from build123d import *

# Parameters (mm, degrees)
SKETCH1_R           = 6.35
BOSS_EXTRUDE1_DEPTH = 17.5
CUT_EXTRUDE1_DEPTH  = 12.9
CHAMFER1_SIZE       = 2
SKETCH4_R           = 3.5
BOSS_EXTRUDE2_DEPTH = 25
SKETCH8_R           = 1.625
CUT_EXTRUDE4_DEPTH  = 30
SKETCH7_R           = 2.2
CUT_EXTRUDE3_DEPTH  = 4.5
SKETCH9_R           = 4
SKETCH9_R_2         = 1.625
BOSS_EXTRUDE3_DEPTH = 5
SKETCH11_R          = 2.75
CUT_EXTRUDE5_DEPTH  = 3
SKETCH12_R          = 1.625
CUT_EXTRUDE6_DEPTH  = 101.436547133
CUT_EXTRUDE8_REACH  = 100.805
SKETCH15_W          = 2
SKETCH15_H          = 32.561115391
SKETCH15_H_2        = 13.634806385
SKETCH16_W          = 2
SKETCH16_H          = 5.291502622
CUT_EXTRUDE9_DEPTH  = 20
CUT_EXTRUDE10_REACH = 102.437
SKETCH17_R          = 1.5
CUT_EXTRUDE11_REACH = 102.437
SKETCH18_W          = 1.2
SKETCH18_H          = 8
SKETCH19_W          = 20
SKETCH19_H          = 25
BOSS_EXTRUDE4_DEPTH = 7
CUT_EXTRUDE12_DEPTH = 35


with BuildPart() as part:
    # Sketch1 → Boss-Extrude1 (new, symmetric)
    with BuildSketch(Plane(origin=(0, 0, 0), x_dir=(0, 0, -1), z_dir=(1, 0, 0))):
        with BuildLine():
            Line((-75, -17.5), (75, -17.5))
            ThreePointArc((75, -17.5), (91.201851746, -6.614378278), (87.247448714, 12.5))
            Line((87.247448714, 12.5), (-69.247448714, 12.5))
            Line((-69.247448714, 12.5), (-69.247448714, 17.5))
            Line((-69.247448714, 17.5), (-75, 17.5))
            ThreePointArc((-75, 17.5), (-92.5, 0), (-75, -17.5))
        make_face()
        with Locations((-75, 0)):
            Circle(SKETCH1_R, mode=Mode.SUBTRACT)
        with Locations((75, 0)):
            Circle(SKETCH1_R, mode=Mode.SUBTRACT)
    extrude(amount=BOSS_EXTRUDE1_DEPTH, both=True)

    # Sketch3 → Cut-Extrude1 (cut, symmetric)
    with BuildSketch(Plane(origin=(0, 0, 0), x_dir=(0, 0, -1), z_dir=(1, 0, 0))):
        with BuildLine():
            Line((-55, -12.5), (75, -12.5))
            ThreePointArc((75, -12.5), (86.858541226, -3.952847075), (82.5, 10))
            Line((82.5, 10), (82.5, 17.5))
            Line((82.5, 17.5), (-92.5, 17.5))
            Line((-92.5, 17.5), (-92.5, -17.5))
            Line((-92.5, -17.5), (-55, -17.5))
            Line((-55, -17.5), (-55, -12.5))
        make_face()
    extrude(amount=CUT_EXTRUDE1_DEPTH, both=True, mode=Mode.SUBTRACT)

    # Chamfer1
    chamfer1_edges = [part.edges().sort_by_distance(p)[0] for p in [
        (17.5, -6.614378278, -91.201851746),
        (17.5, 17.5, 72.123724357),
        (0, -12.5, 55),
        (17.5, 0, 92.5),
        (-17.5, 17.5, 72.123724357),
        (-17.5, -6.614378278, -91.201851746),
        (-17.5, -17.5, 0),
        (-17.5, 0, 92.5),
        (17.5, -17.5, 0),
    ]]
    chamfer(chamfer1_edges, length=CHAMFER1_SIZE)

    # Sketch4 → Boss-Extrude2 (add)
    with BuildSketch(Plane(origin=(0, -12.5, 0), x_dir=(1, 0, 0), z_dir=(0, 1, 0))):
        with Locations((-9.9, 62.5)):
            Circle(SKETCH4_R)
        with Locations((-9.9, 26.333333333)):
            Circle(SKETCH4_R)
        with Locations((-9.9, -9.833333333)):
            Circle(SKETCH4_R)
        with Locations((-9.9, -46)):
            Circle(SKETCH4_R)
    boss_extrude2 = extrude(amount=BOSS_EXTRUDE2_DEPTH)

    # Sketch8 → Cut-Extrude4 (cut)
    with BuildSketch(Plane(origin=(0, 12.5, 0), x_dir=(1, 0, 0), z_dir=(0, 1, 0))):
        with Locations(Location((-9.9, 62.5, 0), (0, 0, 270))):
            Circle(SKETCH8_R)
        with Locations(Location((-9.9, 26.333333333, 0), (0, 0, 270))):
            Circle(SKETCH8_R)
        with Locations(Location((-9.9, -9.833333333, 0), (0, 0, 270))):
            Circle(SKETCH8_R)
        with Locations(Location((-9.9, -46, 0), (0, 0, 270))):
            Circle(SKETCH8_R)
    cut_extrude4 = extrude(amount=-CUT_EXTRUDE4_DEPTH, mode=Mode.SUBTRACT)

    # Sketch7 → Cut-Extrude3 (cut)
    with BuildSketch(Plane.XZ.offset(17.5)):
        with Locations(Location((-9.9, 46, 0), (0, 0, 270))):
            Circle(SKETCH7_R)
        with Locations(Location((-9.9, 9.833333333, 0), (0, 0, 270))):
            Circle(SKETCH7_R)
        with Locations(Location((-9.9, -26.333333333, 0), (0, 0, 270))):
            Circle(SKETCH7_R)
        with Locations(Location((-9.9, -62.5, 0), (0, 0, 270))):
            Circle(SKETCH7_R)
    cut_extrude3 = extrude(amount=-CUT_EXTRUDE3_DEPTH, mode=Mode.SUBTRACT)

    # Sketch9 → Boss-Extrude3 (add, symmetric)
    with BuildSketch(Plane(origin=(0, -12.5, 0), x_dir=(1, 0, 0), z_dir=(0, 1, 0))):
        with Locations((-9.9, 8.25)):
            Circle(SKETCH9_R)
        with Locations(Location((-9.9, 8.25, 0), (0, 0, 270))):
            Circle(SKETCH9_R_2, mode=Mode.SUBTRACT)
    boss_extrude3 = extrude(amount=BOSS_EXTRUDE3_DEPTH, both=True)

    # Sketch11 → Cut-Extrude5 (cut)
    with BuildSketch(Plane.XZ.offset(17.5)):
        with Locations(Location((-9.9, -8.25, 0), (0, 0, 270))):
            Circle(SKETCH11_R)
    cut_extrude5 = extrude(amount=-CUT_EXTRUDE5_DEPTH, mode=Mode.SUBTRACT)

    # Mirror1: Boss-Extrude2, Cut-Extrude4, Cut-Extrude3, Boss-Extrude3, Cut-Extrude5 across plane
    add(boss_extrude2.mirror(Plane(origin=(0, 0, 0), x_dir=(0, 0, 1), z_dir=(1, 0, 0))))
    add(cut_extrude4.mirror(Plane(origin=(0, 0, 0), x_dir=(0, 0, 1), z_dir=(1, 0, 0))), mode=Mode.SUBTRACT)
    add(cut_extrude3.mirror(Plane(origin=(0, 0, 0), x_dir=(0, 0, 1), z_dir=(1, 0, 0))), mode=Mode.SUBTRACT)
    add(boss_extrude3.mirror(Plane(origin=(0, 0, 0), x_dir=(0, 0, 1), z_dir=(1, 0, 0))))
    add(cut_extrude5.mirror(Plane(origin=(0, 0, 0), x_dir=(0, 0, 1), z_dir=(1, 0, 0))), mode=Mode.SUBTRACT)

    # Sketch12 → Cut-Extrude6 (cut, symmetric)
    with BuildSketch(Plane.XZ.offset(17.5)):
        with Locations(Location((9.9, -8.25, 0), (0, 0, 90))):
            Circle(SKETCH12_R)
    cut_extrude6 = extrude(amount=CUT_EXTRUDE6_DEPTH, both=True, mode=Mode.SUBTRACT)

    # Cut-Extrude8: up to this face of the body (flat: up to its plane)
    cut_extrude8_end = Plane(part.part.faces().sort_by_distance((0, -12.5, -11.369745073))[0])
    # Sketch15 → Cut-Extrude8 (cut, up to the picked face)
    with BuildSketch(Plane(origin=(0, 12.5, 0), x_dir=(1, 0, 0), z_dir=(0, 1, 0)), mode=Mode.PRIVATE) as cut_extrude8_sk1:
        with Locations((-13.9, 44.416666667)):
            Rectangle(SKETCH15_W, SKETCH15_H)
    cut_extrude8_tool1 = split(extrude(cut_extrude8_sk1.sketch, amount=-CUT_EXTRUDE8_REACH, mode=Mode.PRIVATE), bisect_by=cut_extrude8_end, keep=Keep.BOTH, mode=Mode.PRIVATE)
    # Sketch15 → Cut-Extrude8 (cut, up to the picked face)
    with BuildSketch(Plane(origin=(0, 12.5, 0), x_dir=(1, 0, 0), z_dir=(0, 1, 0)), mode=Mode.PRIVATE) as cut_extrude8_sk2:
        with Locations((-13.9, 17.713154504)):
            Rectangle(SKETCH15_W, SKETCH15_H_2)
    cut_extrude8_tool2 = split(extrude(cut_extrude8_sk2.sketch, amount=-CUT_EXTRUDE8_REACH, mode=Mode.PRIVATE), bisect_by=cut_extrude8_end, keep=Keep.BOTH, mode=Mode.PRIVATE)
    # Sketch15 → Cut-Extrude8 (cut, up to the picked face)
    with BuildSketch(Plane(origin=(0, 12.5, 0), x_dir=(1, 0, 0), z_dir=(0, 1, 0)), mode=Mode.PRIVATE) as cut_extrude8_sk3:
        with Locations((-13.9, -1.213154504)):
            Rectangle(SKETCH15_W, SKETCH15_H_2)
    cut_extrude8_tool3 = split(extrude(cut_extrude8_sk3.sketch, amount=-CUT_EXTRUDE8_REACH, mode=Mode.PRIVATE), bisect_by=cut_extrude8_end, keep=Keep.BOTH, mode=Mode.PRIVATE)
    # Sketch15 → Cut-Extrude8 (cut, up to the picked face)
    with BuildSketch(Plane(origin=(0, 12.5, 0), x_dir=(1, 0, 0), z_dir=(0, 1, 0)), mode=Mode.PRIVATE) as cut_extrude8_sk4:
        with Locations((-13.9, -27.916666666)):
            Rectangle(SKETCH15_W, SKETCH15_H)
    cut_extrude8_tool4 = split(extrude(cut_extrude8_sk4.sketch, amount=-CUT_EXTRUDE8_REACH, mode=Mode.PRIVATE), bisect_by=cut_extrude8_end, keep=Keep.BOTH, mode=Mode.PRIVATE)
    cut_extrude8_1 = cut_extrude8_tool1.solids().sort_by(Axis((-13.9, 12.5, -44.416667), (0, -1, 0)))[0]
    add(cut_extrude8_1, mode=Mode.SUBTRACT)
    cut_extrude8_2 = cut_extrude8_tool2.solids().sort_by(Axis((-13.9, 12.5, -17.713155), (0, -1, 0)))[0]
    add(cut_extrude8_2, mode=Mode.SUBTRACT)
    cut_extrude8_3 = cut_extrude8_tool3.solids().sort_by(Axis((-13.9, 12.5, 1.213155), (0, -1, 0)))[0]
    add(cut_extrude8_3, mode=Mode.SUBTRACT)
    cut_extrude8_4 = cut_extrude8_tool4.solids().sort_by(Axis((-13.9, 12.5, 27.916667), (0, -1, 0)))[0]
    add(cut_extrude8_4, mode=Mode.SUBTRACT)
    cut_extrude8 = cut_extrude8_1 + cut_extrude8_2 + cut_extrude8_3 + cut_extrude8_4  # Cut-Extrude8 as one shape, for the pattern or mirror that repeats it

    # Sketch16 → Cut-Extrude9 (cut)
    with BuildSketch(Plane(origin=(0, 12.5, 0), x_dir=(1, 0, 0), z_dir=(0, 1, 0))):
        with Locations((-13.9, 8.25)):
            Rectangle(SKETCH16_W, SKETCH16_H)
    cut_extrude9 = extrude(amount=-CUT_EXTRUDE9_DEPTH, mode=Mode.SUBTRACT)

    # Mirror2: Cut-Extrude6, Cut-Extrude8, Cut-Extrude9 across plane
    add(cut_extrude6.mirror(Plane(origin=(0, 0, 0), x_dir=(0, 0, 1), z_dir=(1, 0, 0))), mode=Mode.SUBTRACT)
    add(cut_extrude8.mirror(Plane(origin=(0, 0, 0), x_dir=(0, 0, 1), z_dir=(1, 0, 0))), mode=Mode.SUBTRACT)
    add(cut_extrude9.mirror(Plane(origin=(0, 0, 0), x_dir=(0, 0, 1), z_dir=(1, 0, 0))), mode=Mode.SUBTRACT)

    # Cut-Extrude10: up to this face of the body (flat: up to its plane)
    cut_extrude10_end = Plane(part.part.faces().sort_by_distance((-17.5, -1.343633732, 0.577395586))[0])
    # Sketch17 → Cut-Extrude10 (cut, up to the picked face)
    with BuildSketch(Plane(origin=(17.5, 0, 0), x_dir=(0, 0, -1), z_dir=(1, 0, 0)), mode=Mode.PRIVATE) as cut_extrude10_sk1:
        with Locations((39, 8)):
            Circle(SKETCH17_R)
    cut_extrude10_tool1 = split(extrude(cut_extrude10_sk1.sketch, amount=-CUT_EXTRUDE10_REACH, mode=Mode.PRIVATE), bisect_by=cut_extrude10_end, keep=Keep.BOTH, mode=Mode.PRIVATE)
    add(cut_extrude10_tool1.solids().sort_by(Axis((17.5, 8, -39), (-1, 0, 0)))[0], mode=Mode.SUBTRACT)

    # Cut-Extrude11: up to this face of the body (flat: up to its plane)
    cut_extrude11_end = Plane(part.part.faces().sort_by_distance((17.5, -1.35770743, 0.637008401))[0])
    # Sketch18 → Cut-Extrude11 (cut, up to the picked face)
    with BuildSketch(Plane.ZY.offset(17.5), mode=Mode.PRIVATE) as cut_extrude11_sk1:
        with Locations((-75, 4)):
            Rectangle(SKETCH18_W, SKETCH18_H)
    cut_extrude11_tool1 = split(extrude(cut_extrude11_sk1.sketch, amount=-CUT_EXTRUDE11_REACH, mode=Mode.PRIVATE), bisect_by=cut_extrude11_end, keep=Keep.BOTH, mode=Mode.PRIVATE)
    cut_extrude11 = cut_extrude11_tool1.solids().sort_by(Axis((-17.5, 4, -75), (1, 0, 0)))[0]
    add(cut_extrude11, mode=Mode.SUBTRACT)

    # Mirror3: Cut-Extrude11 across plane
    add(cut_extrude11.mirror(Plane.XY), mode=Mode.SUBTRACT)

    # Sketch19 → Boss-Extrude4 (add)
    with BuildSketch(Plane.ZY.offset(-12.9)):
        with Locations((-75, 0)):
            Rectangle(SKETCH19_W, SKETCH19_H)
    extrude(amount=BOSS_EXTRUDE4_DEPTH)

    # Sketch20 → Cut-Extrude12 (cut)
    with BuildSketch(Plane.ZY.offset(17.5)):
        with BuildLine():
            Line((-75.6, 6.32158999), (-75.6, 8))
            Line((-75.6, 8), (-74.4, 8))
            Line((-74.4, 8), (-74.4, 6.32158999))
            ThreePointArc((-74.4, 6.32158999), (-75, -6.35), (-75.6, 6.32158999))
        make_face()
    extrude(amount=-CUT_EXTRUDE12_DEPTH, mode=Mode.SUBTRACT)


solid = part.part
Geometry: final body of the model. Coordinates: model frame, mm. A direction names the side the tool comes from. Give positions to 0.01 mm unless a question says otherwise; leave off trailing zeros. Loops run counter-clockwise (first coordinate to the right, second up) from the corner with the lowest first, then second, coordinate; pieces in that order, holes last. Notation, with made-up numbers: M 12,42.25 L 45,42.25 A19 ccw 45,56.25 Z; hole C 60,45 d6. An arc over 180 degrees is marked long. Put each result on its own line as item: value. Start each with the question number.
1) Cut plane C-C (z = 19). Output: boundary loops of the cut face in (x, y), then the cut area to 3 significant figures.
2) Pull-direction query (X, two-part tool) for faces 4 (the cylindrical face through (0.22, -6.88, -91.09)), 5 (the conical face through (-17, 0, 91)), 6 (the cylindrical face through (6.402, -0.175, 9.961)); classes: pulls with the +X half, pulls with the -X half, needs draft (parallel to the pull), parting line crosses it, or undercut.
3) Cut plane A-A (z = -8.25). Give the number of separate pieces and of enclosed holes in the cut face, then the cut area to 4 significant figures.
4) Contact query for flat-ended pins moving along their axis: pin 1 (1.8 mm diameter, centred on x = 15.5, y = 7.5, fed in from -Z); pin 2 (3 mm diameter, centred on x = 1, y = 3.5, fed in from +Z); pin 3 (1 mm diameter, centred on x = 14, y = 3, fed in from -Z). Output: stop coordinate, or through.
5) Ray query, line 1 along Z through (x, y) = (-12, 1.5); line 2 along X through (y, z) = (2, -52); line 3 along X through (y, z) = (1, -26.5). Return the intervals inside material, ascending.
6) Access query for faces 1 (the cylindrical face through (-6.402, -0.175, 9.961)), 2 (the cylindrical face through (14.218, 0.385, 92.496)), 3 (the cylindrical face through (10.74, -15.28, 7.8)). Directions: +Z, -Z, +X, -X, +Y, -Y. A direction counts if a zero-diameter tool reaches every point of the face in a straight line with its end or side. Return the directions, or none.
7) Cut plane D-D (z = -62.5). Output: boundary loops of the cut face in (x, y) (3 decimals), then the cut area to 3 significant figures.
Verdict:
1. outline: M -17.5,-15.5 L -15.5,-17.5 L 15.5,-17.5 L 17.5,-15.5 L 17.5,12.5 L 14.9,12.5 L 14.9,-12.5 L -14.9,-12.5 L -14.9,12.5 L -17.5,12.5 Z
1. area: 301 mm2
2. face 4: needs draft
2. face 5: pulls with the -X half
2. face 6: undercut
3. separate pieces: 3
3. enclosed holes: 0
3. area: 312.5 mm2
4. pin 1: z = -91.21
4. pin 2: z = -86.46
4. pin 3: z = -92.32
5. line 1: -92.44 to -87.41, -65.3 to -59.7, -29.13 to -23.53, 7.03 to 12.63, 43.2 to 48.8
5. line 2: -17.5 to -14.9, 14.9 to 17.5
5. line 3: -17.5 to -11.52, -8.28 to -6.4, 6.4 to 8.28, 11.52 to 17.5
6. face 1: +Y
6. face 2: +Z, +X, -X
6. face 3: -Y
7. outline: M -17.5,-15.5 L -15.5,-17.5 L -12.1,-17.5 L -12.1,-13 L -11.525,-13 L -11.525,12.5 L -17.5,12.5 Z; M -8.275,-13 L -7.7,-13 L -7.7,-17.5 L 7.7,-17.5 L 7.7,-13 L 8.275,-13 L 8.275,12.5 L 6.4,12.5 L 6.4,-12.5 L -6.4,-12.5 L -6.4,12.5 L -8.275,12.5 Z; M 11.525,-13 L 12.1,-13 L 12.1,-17.5 L 15.5,-17.5 L 17.5,-15.5 L 17.5,12.5 L 11.525,12.5 Z
7. area: 521 mm2
